Verification items for the finished model (mm, model axes). A direction names the side the tool comes from. Round coordinates to 2 decimals unless told otherwise and drop trailing zeros. Write each loop counter-clockwise with the first axis right and the second up, starting at its lowest first coordinate (ties: lowest second). Pieces come first, ordered by that corner, then holes. Notation, with made-up numbers: M 19.25,67 L 56.25,67 A6 cw 56.25,73 Z; hole C -17,44 d7. An arc over 180 degrees is marked long. One line per item, written item: value. Start each with the question number.
from build123d import *

# Parameters (mm, degrees)
F0_R      = 45
F1_DEPTH  = 417
F2_R      = 40
F3_DEPTH  = 110
F4_R      = 35
F5_DEPTH  = 182
F6_R      = 30
F7_DEPTH  = 80
F8_R      = 50
F9_DEPTH  = 120
F10_R     = 55
F11_DEPTH = 204
F12_R     = 45
F13_DEPTH = 90


with BuildPart() as f1:
    # F0 (on Front) → F1 (new body)
    with BuildSketch(Plane.XZ):
        Circle(F0_R)
    extrude(amount=-F1_DEPTH)

    # F2 (on face) → F3 (join)
    with BuildSketch(Plane(origin=(0, 417, 0), x_dir=(-1, 0, 0), z_dir=(0, 1, 0))):
        Circle(F2_R)
    extrude(amount=F3_DEPTH)

    # F4 (on face) → F5 (join)
    with BuildSketch(Plane(origin=(0, 527, 0), x_dir=(-1, 0, 0), z_dir=(0, 1, 0))):
        Circle(F4_R)
    extrude(amount=F5_DEPTH)

    # F6 (on face) → F7 (join)
    with BuildSketch(Plane(origin=(0, 709, 0), x_dir=(-1, 0, 0), z_dir=(0, 1, 0))):
        Circle(F6_R)
    extrude(amount=F7_DEPTH)

    # F8 (on face) → F9 (join)
    with BuildSketch(Plane.XZ):
        Circle(F8_R)
    extrude(amount=F9_DEPTH)

    # F10 (on face) → F11 (join)
    with BuildSketch(Plane.XZ.offset(120)):
        Circle(F10_R)
    extrude(amount=F11_DEPTH)

    # F12 (on face) → F13 (join)
    with BuildSketch(Plane.XZ.offset(324)):
        Circle(F12_R)
    extrude(amount=F13_DEPTH)


solid = f1.part
1) Access from +Z, -Z, +X, -X, +Y, -Y to the whole of each face (thin tool, end or side, straight path). Record for faces 1 (the flat face through (-21, -324, -40)), 2 (the cylindrical face through (-11.923, -220.572, -53.692)), 3 (the cylindrical face through (20.765, 205.581, -39.923)).
2) Cross-section at B-B (x = 16). Record the boundary of the cut face in (y, z).
3) Cross-section at A-A (z = 0). Record the boundary of the cut face in (x, y).
4) Cross-section at D-D (y = 581). Record the boundary of the cut face in (x, z), then the cut area to 3 significant figures.
5) Gauge pin test, flat ends, axial feed: pin 1 Ø8 at (y, z) = (655, 20) entering from +X; pin 2 Ø4 at (y, z) = (-253, 35) entering from -X; pin 3 Ø8 at (y, z) = (177.5, 33) entering from -X. Record the tip position at first contact, or that the pin passes through.
6) Cross-section at C-C (y = 281). Record the boundary of the cut face in (x, z).
7) Thickness scan on line 1 (X direction, y = 576, z = 4); line 2 (Y direction, x = -23.5, z = 43.5); line 3 (Y direction, x = 23.5, z = 26). Record the ranges inside material, lowest first.
Results below:
1. face 1: -Y
1. face 2: +Y, -Y
1. face 3: +Y
2. outline: M -414,-42.06 L -324,-42.06 L -324,-52.62 L -120,-52.62 L -120,-47.37 L 0,-47.37 L 0,-42.06 L 417,-42.06 L 417,-36.66 L 527,-36.66 L 527,-31.13 L 709,-31.13 L 709,-25.38 L 789,-25.38 L 789,25.38 L 709,25.38 L 709,31.13 L 527,31.13 L 527,36.66 L 417,36.66 L 417,42.06 L 0,42.06 L 0,47.37 L -120,47.37 L -120,52.62 L -324,52.62 L -324,42.06 L -414,42.06 Z
3. outline: M -55,-324 L -45,-324 L -45,-414 L 45,-414 L 45,-324 L 55,-324 L 55,-120 L 50,-120 L 50,0 L 45,0 L 45,417 L 40,417 L 40,527 L 35,527 L 35,709 L 30,709 L 30,789 L -30,789 L -30,709 L -35,709 L -35,527 L -40,527 L -40,417 L -45,417 L -45,0 L -50,0 L -50,-120 L -55,-120 Z
4. outline: C 0,0 d70
4. area: 3,850 mm²
5. pin 1: stops at x = 31.13
5. pin 2: stops at x = -44
5. pin 3: stops at x = -34.41
6. outline: C 0,0 d90
7. line 1: x = -34.77 to 34.77
7. line 2: y = -324 to 0
7. line 3: y = -414 to 527
